```python
from build123d import *

# Parameters (mm, degrees)
SKETCH2_R           = 32.5
BOSS_EXTRUDE1_DEPTH = 60
CUT_REVOLVE1_ANGLE  = 180
CUT_EXTRUDE1_REACH  = 12
SKETCH5_W           = 97.630906447
SKETCH5_H           = 85.301230118
SKETCH7_R           = 30
CUT_EXTRUDE3_DEPTH  = 39
SKETCH8_R           = 1
BOSS_EXTRUDE2_DEPTH = 5
SKETCH9_R           = 5
CUT_EXTRUDE4_DEPTH  = 1


with BuildPart() as part:
    # Sketch2 → Boss-Extrude1 (new body)
    with BuildSketch(Plane.XY):
        Circle(SKETCH2_R)
    extrude(amount=BOSS_EXTRUDE1_DEPTH)

    # Sketch4 → Cut-Revolve1 (revolve, cut)
    with BuildSketch(Plane.XY.offset(55)):
        with BuildLine():
            Line((-16.25, 0), (16.25, 0))
            ThreePointArc((16.25, 0), (0, 16.25), (-16.25, 0))
        make_face()
    revolve(axis=Axis((-16.25, 0, 55), (-1, 0, 0)), revolution_arc=CUT_REVOLVE1_ANGLE, mode=Mode.SUBTRACT)

    # Sketch5 → Cut-Extrude1 (cut, up to next)
    with BuildSketch(Plane.XY.offset(50), mode=Mode.PRIVATE) as cut_extrude1_sk1:
        with Locations((-1.59772985, 0.365427289)):
            Rectangle(SKETCH5_W, SKETCH5_H)
    cut_extrude1_tool1 = extrude(cut_extrude1_sk1.sketch, amount=CUT_EXTRUDE1_REACH, mode=Mode.PRIVATE) & part.part
    add(cut_extrude1_tool1.solids().sort_by_distance((-1.59773, 0.365427, 50))[0], mode=Mode.SUBTRACT)

    # Sketch7 → Cut-Extrude3 (cut)
    with BuildSketch(Plane(origin=(0, 0, 0), x_dir=(-1, 0, 0), z_dir=(0, 0, -1))):
        Circle(SKETCH7_R)
    extrude(amount=-CUT_EXTRUDE3_DEPTH, mode=Mode.SUBTRACT)

    # Sketch8 → Boss-Extrude2 (add)
    with BuildSketch(Plane(origin=(0, 0, 39), x_dir=(-1, 0, 0), z_dir=(0, 0, -1))):
        with Locations((17.5, -9)):
            Circle(SKETCH8_R)
        with Locations((-17.5, -9)):
            Circle(SKETCH8_R)
    extrude(amount=BOSS_EXTRUDE2_DEPTH)

    # Sketch9 → Cut-Extrude4 (cut)
    with BuildSketch(Plane(origin=(0, 0, 39), x_dir=(-1, 0, 0), z_dir=(0, 0, -1))):
        Circle(SKETCH9_R)
    extrude(amount=-CUT_EXTRUDE4_DEPTH, mode=Mode.SUBTRACT)


solid = part.part
```
Verification items for the finished model (mm, model axes). A direction names the side the tool comes from. Round coordinates to 2 decimals unless told otherwise and drop trailing zeros. Order: outer loops, then holes, each group sorted by start corner. A loop starts at its lowest first (then second) coordinate and runs counter-clockwise, first axis right, second up. Notation, with made-up numbers: (3, 5) - (26, 5) arc R15 cw to (26, 9) - close; hole circle Ø2 at (62.5, -14). An arc over 180 degrees is marked (long way). Use CSV: the item, a comma, the result in double quotes.
(1) Section check D-D on y = 14. Record the boundary of the cut face in (x, z).
Entries:
outline,"(-29.33, 0) - (-26.53, 0) - (-26.53, 39) - (26.53, 39) - (26.53, 0) - (29.33, 0) - (29.33, 50) - (6.56, 50) arc R8.25 cw to (-6.56, 50) - (-29.33, 50) - close"
(2) Section check A-A on x = 0. Record the boundary of the cut face in (y, z).
Entries:
outline,"(-32.5, 0) - (-30, 0) - (-30, 39) - (-5, 39) - (-5, 39.54) arc R16.25 cw to (-15.46, 50) - (-32.5, 50) - close; (5, 39) - (30, 39) - (30, 0) - (32.5, 0) - (32.5, 50) - (15.46, 50) arc R16.25 cw to (5, 39.54) - close"
(3) Thickness scan on probe 1 along Y at (x, z) = (0, 28); probe 2 along X at (y, z) = (-1, 5); probe 3 along Y at (x, z) = (0, 39.4). Record the ranges inside material, lowest first. Write a range as from..to.
Entries:
probe 1,"-32.5..-30, 30..32.5"
probe 2,"-32.48..-29.98, 29.98..32.48"
probe 3,"-32.5..-5, 5..32.5"
(4) Gauge pin test, flat ends, axial feed: pin 1 Ø1.5 at (y, z) = (13, 14) entering from -X; pin 2 Ø2 at (x, y) = (18, -8.5) entering from -Z; pin 3 Ø10 at (y, z) = (-9.5, 12.5) entering from -X. Record the tip position at first contact, or that the pin passes through.
Entries:
pin 1,"x = -30.1"
pin 2,"z = 34"
pin 3,"x = -32.19"
(5) Section check B-B on z = 38. Record the boundary of the cut face in (x, y).
Entries:
outline,"circle Ø65 at (0, 0); circle Ø2 at (-17.5, -9); circle Ø2 at (17.5, -9); hole circle Ø60 at (0, 0)"
(6) Mould release check, pull along Y, two halves, no side actions. Record for faces 1 (the face through (9, -29, 0)), 2 (the face through (31, 9.76, 24.65)), 3 (the face through (18, -9, 34)): released by +Y, released by -Y, zero draft, split by the parting line, or undercut.
Entries:
face 1,"zero draft"
face 2,"split by the parting line"
face 3,"undercut"
(7) Access from +Z, -Z, +X, -X, +Y, -Y to the whole of each face (thin tool, end or side, straight path). Record for faces 4 (the face through (-18.04, -8.16, 36.53)), 5 (the face through (14, -7, 50)).
Entries:
face 4,"-Z"
face 5,"+Z, +X, -X, +Y, -Y"
